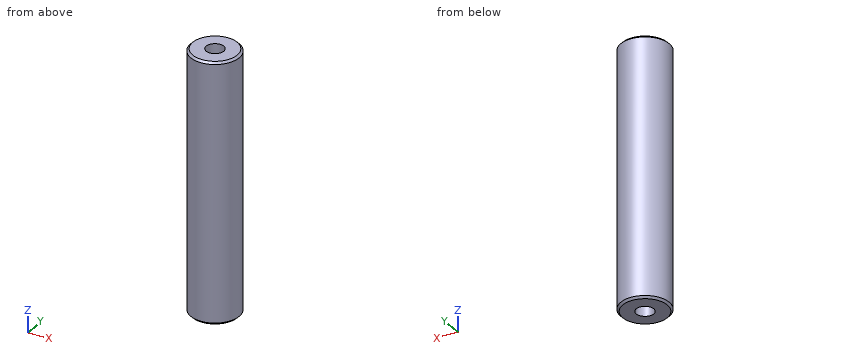
```python
from build123d import *

# Parameters (mm, degrees)
SKETCH1_R                               = 4.7625
BOSS_EXTRUDE1_DEPTH                     = 25.4
TAP_DRILL_FOR_8_32_TAP1_D               = 3.4544
TAP_DRILL_FOR_8_32_TAP1_DEPTH           = 6.35
TAP_DRILL_FOR_8_32_TAP1_TIP             = 1.037806461
TAP_DRILL_FOR_8_32_TAP1_ON_FACE_2_D     = 3.4544
TAP_DRILL_FOR_8_32_TAP1_ON_FACE_2_DEPTH = 6.35
TAP_DRILL_FOR_8_32_TAP1_ON_FACE_2_TIP   = 1.037806461
CHAMFER1_SIZE                           = 0.396875


with BuildPart() as part:
    # Sketch1 → Boss-Extrude1 (new, symmetric)
    with BuildSketch(Plane.XY):
        Circle(SKETCH1_R)
    extrude(amount=BOSS_EXTRUDE1_DEPTH, both=True)

    # Tap Drill for #8-32 Tap1
    with Locations(Plane.XY.offset(25.4)):
        with Locations((0, 0)):
            Hole(TAP_DRILL_FOR_8_32_TAP1_D / 2, depth=TAP_DRILL_FOR_8_32_TAP1_DEPTH)
            with Locations((0, 0, -(TAP_DRILL_FOR_8_32_TAP1_DEPTH + TAP_DRILL_FOR_8_32_TAP1_TIP / 2))):  # 118° drill point
                Cone(0, TAP_DRILL_FOR_8_32_TAP1_D / 2, TAP_DRILL_FOR_8_32_TAP1_TIP, mode=Mode.SUBTRACT)

    # Tap Drill for #8-32 Tap1 on face 2
    with Locations(Plane(origin=(0, 0, -25.4), x_dir=(-1, 0, 0), z_dir=(0, 0, -1))):
        with Locations((0, 0)):
            Hole(TAP_DRILL_FOR_8_32_TAP1_ON_FACE_2_D / 2, depth=TAP_DRILL_FOR_8_32_TAP1_ON_FACE_2_DEPTH)
            with Locations((0, 0, -(TAP_DRILL_FOR_8_32_TAP1_ON_FACE_2_DEPTH + TAP_DRILL_FOR_8_32_TAP1_ON_FACE_2_TIP / 2))):  # 118° drill point
                Cone(0, TAP_DRILL_FOR_8_32_TAP1_ON_FACE_2_D / 2, TAP_DRILL_FOR_8_32_TAP1_ON_FACE_2_TIP, mode=Mode.SUBTRACT)

    # Chamfer1
    chamfer1_edges = [part.edges().sort_by_distance(p)[0] for p in [
        (-4.7625, 0, -25.4),
        (-4.7625, 0, 25.4),
    ]]
    chamfer(chamfer1_edges, length=CHAMFER1_SIZE)


solid = part.part
```
CAD build for the part. Positions are in the model's coordinates, mm. Round coordinates to 2 decimals unless told otherwise and drop trailing zeros. Order: outer loops, then holes, each group sorted by start corner. A loop starts at its lowest first (then second) coordinate and runs counter-clockwise, first axis right, second up.
Q1. Wall check: L1, parallel to Y at x = 0, z = 20.75; L2, parallel to Y at x = -0.25, z = 3.5; L3, parallel to Z at x = -4.25, y = 1.25. Give the ranges that are in metal, low to high.
Q2. Slice it at A-A (z = 13). Write the cut outline in (x, y) (1 decimal).
Q3. Drop flat-ended pins along their axis: pin 1 (2 mm diameter, centred on x = 0, y = 0, fed in from -Z); pin 2 (1 mm diameter, centred on x = -1.5, z = -0.5, fed in from -Y); pin 3 (1 mm diameter, centred on x = 1, y = 0, fed in from -Z). Give the stop position or say it passes through.
Results below:
1. L1: y = -4.76 to -1.73, 1.73 to 4.76
1. L2: y = -4.76 to 4.76
1. L3: z = -25.34 to 25.34
2. outline: circle Ø9.5 at (0, 0)
3. pin 1: stops at z = -18.61
3. pin 2: stops at y = -4.66
3. pin 3: stops at z = -18.91
